```python
from build123d import *

# Parameters (mm, degrees)
BASPROSKE_W         = 10
BASPROSKE_H         = 6
TOOTHCUT_DEPTH      = 14.114877049
TEETHCUTS_COUNT     = 10
TEETHCUTS_ANGLE     = 324
BORSKE_R            = 2.5
BORE_DEPTH          = 50.0000508
SKETCH1_R           = 2.5
BOSS_EXTRUDE1_DEPTH = 10
CUT_EXTRUDE2_DEPTH  = 10
CUT_EXTRUDE4_DEPTH  = 12.8


with BuildPart() as part:
    # BasProSke → Base-Revolve (revolve)
    with BuildSketch(Plane(origin=(0, 0, 0), x_dir=(1, 0, 0), z_dir=(0, 1, 0)), mode=Mode.PRIVATE) as base_revolve_sk:
        with Locations((5, 3)):
            Rectangle(BASPROSKE_W, BASPROSKE_H)
    revolve(base_revolve_sk.sketch.rotate(Axis((-10, 0, 0), (1, 0, 0)), 180), axis=Axis((-10, 0, 0), (1, 0, 0)))

    # TooCutSke → ToothCut (cut, through all)
    with BuildSketch(Plane(origin=(0, 0, 0), x_dir=(0, 0, -1), z_dir=(1, 0, 0))):
        with BuildLine():
            ThreePointArc((0.59278292, 3.701838653), (0, 3.749), (-0.59278292, 3.701838653))
            ThreePointArc((-0.59278292, 3.701838653), (-0.846593509, 4.924114224), (-1.775771316, 5.757784417))
            ThreePointArc((-1.775771316, 5.757784417), (0, 6.0254), (1.775771316, 5.757784417))
            ThreePointArc((1.775771316, 5.757784417), (0.846593509, 4.924114224), (0.59278292, 3.701838653))
        make_face()
    toothcut = extrude(amount=TOOTHCUT_DEPTH, mode=Mode.SUBTRACT)

    # TeethCuts: ToothCut ×10 about axis
    teethcuts_axis = Axis((-10, 0, 0), (1, 0, 0))
    for i in range(1, TEETHCUTS_COUNT):
        add(toothcut.rotate(teethcuts_axis, i * TEETHCUTS_ANGLE / (TEETHCUTS_COUNT - 1)), mode=Mode.SUBTRACT)

    # BorSke → Bore (cut, symmetric)
    with BuildSketch(Plane(origin=(0, 0, 0), x_dir=(0, 0, -1), z_dir=(1, 0, 0))):
        with Locations(Location((0, 0, 0), (0, 0, 180))):
            Circle(BORSKE_R)
    extrude(amount=BORE_DEPTH, both=True, mode=Mode.SUBTRACT)

    # Sketch1 → Boss-Extrude1 (add)
    with BuildSketch(Plane(origin=(10, 0, 0), x_dir=(0, 0, -1), z_dir=(1, 0, 0))):
        Circle(SKETCH1_R)
    extrude(amount=-BOSS_EXTRUDE1_DEPTH)

    # Sketch2 → Cut-Extrude2 (cut)
    with BuildSketch(Plane.ZY):
        with BuildLine():
            Line((1.187434209, 2.2), (-1.187434209, 2.2))
            ThreePointArc((-1.187434209, 2.2), (-1.280900948, -2.146926352), (2.5, 0))
            ThreePointArc((2.5, 0), (2.146926352, 1.280900948), (1.187434209, 2.2))
        make_face()
    extrude(amount=-CUT_EXTRUDE2_DEPTH, mode=Mode.SUBTRACT)

    # Sketch3 → Cut-Extrude4 (cut)
    with BuildSketch(Plane.ZY):
        with BuildLine():
            ThreePointArc((-1.385640646, 2.2), (0, -2.6), (1.385640646, 2.2))
            Line((1.385640646, 2.2), (-1.385640646, 2.2))
        make_face()
    extrude(amount=-CUT_EXTRUDE4_DEPTH, mode=Mode.SUBTRACT)


solid = part.part
```
Part model, mm, in its own coordinate system. Round coordinates to 2 decimals unless told otherwise and drop trailing zeros. Order: outer loops, then holes, each group sorted by start corner. A loop starts at its lowest first (then second) coordinate and runs counter-clockwise, first axis right, second up. Notation, with made-up numbers: M -27,85 L 27,85 A13 ccw 27,89 Z; hole C 47.25,11.25 d8. An arc over 180 degrees is marked long. Put each result on its own line as item: value. Start each with the question number.
1. Slice it at B-B on z = 5.25. List the corners of the cut face in (x, y).
2. Two-plate mould, pull along Z, no slides. Class faces 1 (the face through (4.93, 3.485, -3.578)), 2 (the face through (10, 0, 3)): +Z half, -Z half, draft (parallel to the pull), parting line (faces both ways), or undercut.
3. Slice it at A-A on z = 0. List the corners of the cut face in (x, y).
4. Drill centre lines: probe 1 along Y at (x, z) = (5.5, 4.5); probe 2 along Z at (x, y) = (2.5, -3); probe 3 along Y at (x, z) = (0.5, -4). Where is each one in solid material? Low to high. Write a range as [from, to].
5. Drop flat-ended pins along their axis: pin 1 (2 mm diameter, centred on x = 4.5, z = 0, fed in from -Y); pin 2 (3 mm diameter, centred on x = 7, z = -3.5, fed in from +Y); pin 3 (6 mm diameter, centred on x = 9, y = -4.5, fed in from +Z). Give the stop position or say it passes through.
Findings:
1. outline: M 0,-0.63 L 10,-0.63 L 10,0.63 L 0,0.63 Z
2. face 1: undercut
2. face 2: draft
3. outline: M 0,-3.75 L 10,-3.75 L 10,-2.6 L 0,-2.6 Z; M 0,2.2 L 10,2.2 L 10,3.75 L 0,3.75 Z
4. probe 1: [-3.66, -2.42], [-0.76, 0.76], [2.42, 3.66]
4. probe 2: [-4.82, -2.91], [-2.25, 2.25], [2.91, 4.82]
4. probe 3: [-3.62, -1.97], [-0.69, 0.69], [1.97, 3.62]
5. pin 1: y = -5.15
5. pin 2: y = 5.61
5. pin 3: z = 4.92
